Work out the finished part from the listing and answer in its coordinate system (mm). A direction names the side the tool comes from. Coordinates: 2 decimals unless noted, no trailing zeros. Loops run counter-clockwise (first coordinate to the right, second up) from the corner with the lowest first, then second, coordinate; pieces in that order, holes last. Notation, with made-up numbers: (42, 43) -> (64, 43) arc R22 ccw to (64, 58) -> close; hole circle Ø9 at (40.25, 80.25). An arc over 180 degrees is marked (long way). Use a Markdown table: item, result.
from build123d import *

# Parameters (mm, degrees)
SKETCH1_R           = 37.5
SKETCH1_R_2         = 2.25
BOSS_EXTRUDE1_DEPTH = 10
CUT_EXTRUDE1_DEPTH  = 4
FILLET1_R           = 3


with BuildPart() as part:
    # Sketch1 → Boss-Extrude1 (new body)
    with BuildSketch(Plane(origin=(0, 0, 0), x_dir=(1, 0, 0), z_dir=(0, 1, 0))):
        Circle(SKETCH1_R)
        with Locations((0, 27.5)):
            Circle(SKETCH1_R_2, mode=Mode.SUBTRACT)
        with Locations((23.815698604, 13.75)):
            Circle(SKETCH1_R_2, mode=Mode.SUBTRACT)
        with Locations((23.815698604, -13.75)):
            Circle(SKETCH1_R_2, mode=Mode.SUBTRACT)
        with Locations((0, -27.5)):
            Circle(SKETCH1_R_2, mode=Mode.SUBTRACT)
        with Locations((-23.815698604, -13.75)):
            Circle(SKETCH1_R_2, mode=Mode.SUBTRACT)
        with Locations((-23.815698604, 13.75)):
            Circle(SKETCH1_R_2, mode=Mode.SUBTRACT)
    extrude(amount=BOSS_EXTRUDE1_DEPTH)

    # Sketch2 → Cut-Extrude1 (cut)
    with BuildSketch(Plane(origin=(0, 10, 0), x_dir=(1, 0, 0), z_dir=(0, 1, 0))):
        with BuildLine():
            Line((12, -5), (12, 0))
            Line((12, 0), (12, 5))
            Line((12, 5), (-37.165171868, 5))
            ThreePointArc((-37.165171868, 5), (-37.5, 0), (-37.165171868, -5))
            Line((-37.165171868, -5), (12, -5))
        make_face()
    extrude(amount=-CUT_EXTRUDE1_DEPTH, mode=Mode.SUBTRACT)

    # Fillet1
    fillet1_edges = [part.edges().sort_by_distance(p)[0] for p in [
        (-12.582585934, 6, -5),
        (12, 6, 0),
        (-12.582585934, 6, 5),
    ]]
    fillet(fillet1_edges, radius=FILLET1_R)


solid = part.part
Q1. Section A-A on x = 0 is taken. Determine the outline of the cut face in (y, z).
Solved:
| item | result |
|---|---|
| outline | (0, -37.5) -> (10, -37.5) -> (10, -29.75) -> (0, -29.75) -> close; (0, -25.25) -> (10, -25.25) -> (10, -5) -> (9, -5) arc R3 cw to (6, -2) -> (6, 2) arc R3 cw to (9, 5) -> (10, 5) -> (10, 25.25) -> (0, 25.25) -> close; (0, 29.75) -> (10, 29.75) -> (10, 37.5) -> (0, 37.5) -> close |
Q2. Section C-C on z = 27.5 is taken. Determine the outline of the cut face in (x, y), and give its area (3 significant figures).
Solved:
| item | result |
|---|---|
| outline | (-25.5, 0) -> (-2.25, 0) -> (-2.25, 10) -> (-25.5, 10) -> close; (2.25, 0) -> (25.5, 0) -> (25.5, 10) -> (2.25, 10) -> close |
| area | 465 mm² |
Q3. Given pin 1 Ø4 at (x, y) = (2.5, 3.5) entering from +Z; pin 2 Ø3.5 at (x, z) = (23.82, 13.75) entering from -Y; pin 3 Ø1.5 at (x, z) = (-17, 2) entering from +Y; pin 4 Ø1.1 at (x, y) = (-22, 9.5) entering from -Z, each flat-ended and moving along its own axis, determine where each tip first touches the part or whether it passes through.
Solved:
| item | result |
|---|---|
| pin 1 | z = 37.5 |
| pin 2 | through |
| pin 3 | y = 6.1 |
| pin 4 | z = -30.76 |
Q4. Consider line 1 (X direction, y = 2.25, z = 13.75); line 2 (Z direction, x = 0, y = 8.25); line 3 (X direction, y = 9.5, z = 13). Determine where each line is inside the solid, lowest interval first. Write a range as [from, to].
Solved:
| item | result |
|---|---|
| line 1 | [-34.89, -26.07], [-21.57, 21.57], [26.07, 34.89] |
| line 2 | [-37.5, -29.75], [-25.25, -4.9], [4.9, 25.25], [29.75, 37.5] |
| line 3 | [-35.17, -25.94], [-21.69, 21.69], [25.94, 35.17] |
Q5. Determine the mould class of faces 3 (the flat face through (-1, 0, -1)), 4 (the cylindrical face through (35.77, 4.93, -11.26)), 5 (the cylindrical face through (-13.07, 6.86, -4.1)) for opening direction Z: pulls with the +Z half, pulls with the -Z half, needs draft (parallel to the pull), parting line crosses it, or undercut.
Solved:
| item | result |
|---|---|
| face 3 | needs draft |
| face 4 | parting line crosses it |
| face 5 | undercut |
Q6. For faces 1 (the cylindrical face through (-0.488, 4.93, 29.696)), 2 (the cylindrical face through (11.438, 7.252, -0.07)), determine the directions among +Z, -Z, +X, -X, +Y, -Y from which every point of the face is accessible in a straight line to the end or side of a thin tool.
Solved:
| item | result |
|---|---|
| face 1 | +Y, -Y |
| face 2 | -X, +Y |
Q7. Section B-B on y = 2.25 is taken. Determine the outline of the cut face in (x, z).
Solved:
| item | result |
|---|---|
| outline | circle Ø75 at (0, 0); hole circle Ø4.5 at (-23.82, -13.75); hole circle Ø4.5 at (-23.82, 13.75); hole circle Ø4.5 at (0, -27.5); hole circle Ø4.5 at (0, 27.5); hole circle Ø4.5 at (23.82, -13.75); hole circle Ø4.5 at (23.82, 13.75) |
Q8. Section D-D on z = -13.75 is taken. Determine the outline of the cut face in (x, y), and give its area (3 significant figures).
Solved:
| item | result |
|---|---|
| outline | (-34.89, 0) -> (-26.07, 0) -> (-26.07, 10) -> (-34.89, 10) -> close; (-21.57, 0) -> (21.57, 0) -> (21.57, 10) -> (-21.57, 10) -> close; (26.07, 0) -> (34.89, 0) -> (34.89, 10) -> (26.07, 10) -> close |
| area | 608 mm² |
